For this review, take the finished solid that the model builds, in its own axes (mm). A direction names the side the tool comes from. Coordinates: 2 decimals unless noted, no trailing zeros. Loops run counter-clockwise (first coordinate to the right, second up) from the corner with the lowest first, then second, coordinate; pieces in that order, holes last.
```python
from build123d import *

# Parameters (mm, degrees)
CLAMP_DEPTH      = 8
SKETCH2_R        = 2.1
SCREW_HOLE_DEPTH = 31.055157627


with BuildPart() as part:
    # Sketch1 → Clamp (new body)
    with BuildSketch(Plane.XY):
        with BuildLine():
            Line((-6.631553363, 7.75), (6.631553363, 7.75))
            ThreePointArc((6.631553363, 7.75), (9.265037623, 4.266037723), (10.2, 0))
            Line((10.2, 0), (10.2, -10.5))
            Line((10.2, -10.5), (22.5, -10.5))
            Line((22.5, -10.5), (22.5, -7.5))
            Line((22.5, -7.5), (13, -7.5))
            Line((13, -7.5), (13, 0))
            ThreePointArc((13, 0), (11.489805152, 6.081478239), (7.310095759, 10.75))
            Line((7.310095759, 10.75), (-7.310095759, 10.75))
            ThreePointArc((-7.310095759, 10.75), (-11.489805152, 6.081478239), (-13, 0))
            Line((-13, 0), (-13, -7.5))
            Line((-13, -7.5), (-22.5, -7.5))
            Line((-22.5, -7.5), (-22.5, -10.5))
            Line((-22.5, -10.5), (-10.2, -10.5))
            Line((-10.2, -10.5), (-10.2, 0))
            ThreePointArc((-10.2, 0), (-9.265037623, 4.266037723), (-6.631553363, 7.75))
        make_face()
    extrude(amount=CLAMP_DEPTH)

    # Sketch2 → Screw Hole (cut, through all)
    with BuildSketch(Plane(origin=(0, -7.5, 0), x_dir=(1, 0, 0), z_dir=(0, 1, 0))):
        with Locations(Location((-17.75, -4, 0), (0, 0, 270))):
            Circle(SKETCH2_R)
        with Locations(Location((17.75, -4, 0), (0, 0, 270))):
            Circle(SKETCH2_R)
    extrude(amount=-SCREW_HOLE_DEPTH, mode=Mode.SUBTRACT)


solid = part.part
```
Q1. The part is to be moulded in two halves that separate along X. For faces 5 (the face through (11.531, 6.003, 3.944)), 6 (the face through (15, -10.5, 4)), 7 (the face through (-9.29, 4.21, 3.94)), say which applies: +X half, -X half, draft (parallel to the pull), parting line (faces both ways), or undercut.
Q2. Consider section C-C (x = -17.75). State the section outline as (y, z) points, then the cut area to 3 significant figures.
Q3. Consider section B-B (y = -6.75). State the section outline as (x, z) points, then the cut area to 3 significant figures.
Q4. Consider section A-A (z = 4). State the section outline as (x, y) points, then the cut area to 3 significant figures.
Q5. Wall thickness on probe 1 along X at (y, z) = (-9.65, 4); probe 2 along X at (y, z) = (-0.5, 5.5); probe 3 along Y at (x, z) = (-13.5, 7): over which ranges is each line inside the solid? List them lowest first.
Q6. Machinability: for faces 1 (the face through (-15.668, -8.979, 3.727)), 2 (the face through (-10.2, -5, 4)), 3 (the face through (13, -4, 4)), 4 (the face through (-15.6, -7.5, 3.1)), which of the approach directions +Z, -Z, +X, -X, +Y, -Y give a long, thin tool a straight path to every point of the face, cutting with its end or side? Answer none if there is none.
Q7. Consider section D-D (z = 7.5). State the section outline as (x, y) points, then the cut area to 3 significant figures.
Q8. For pin 1 Ø2.5 at (x, z) = (0.5, 5) entering from -Y; pin 2 Ø2.5 at (x, z) = (-18.5, 3) entering from +Y; pin 3 Ø1 at (y, z) = (-6.5, 4.5) entering from +X, all flat-tipped, find the tip position at first contact; note any pin that passes through.
Model answer:
1. face 5: +X half
1. face 6: draft
1. face 7: undercut
2. outline: (-10.5, 0) - (-7.5, 0) - (-7.5, 1.9) - (-10.5, 1.9) - close; (-10.5, 6.1) - (-7.5, 6.1) - (-7.5, 8) - (-10.5, 8) - close
2. area: 11.4 mm2
3. outline: (-13, 0) - (-10.2, 0) - (-10.2, 8) - (-13, 8) - close; (10.2, 0) - (13, 0) - (13, 8) - (10.2, 8) - close
3. area: 44.8 mm2
4. outline: (-22.5, -10.5) - (-19.85, -10.5) - (-19.85, -7.5) - (-22.5, -7.5) - close; (-15.65, -10.5) - (-10.2, -10.5) - (-10.2, 0) arc R10.2 cw to (-6.63, 7.75) - (6.63, 7.75) arc R10.2 cw to (10.2, 0) - (10.2, -10.5) - (15.65, -10.5) - (15.65, -7.5) - (13, -7.5) - (13, 0) arc R13 ccw to (7.31, 10.75) - (-7.31, 10.75) arc R13 ccw to (-13, 0) - (-13, -7.5) - (-15.65, -7.5) - close; (19.85, -10.5) - (22.5, -10.5) - (22.5, -7.5) - (19.85, -7.5) - close
4. area: 193 mm2
5. probe 1: x = -22.5 to -19.85, -15.65 to -10.2, 10.2 to 15.65, 19.85 to 22.5
5. probe 2: x = -13 to -10.2, 10.2 to 13
5. probe 3: y = -10.5 to -7.5
6. face 1: +Y, -Y
6. face 2: +Z, -Z, -Y
6. face 3: +Z, -Z, +X, +Y
6. face 4: +Z, -Z, -X, +Y
7. outline: (-22.5, -10.5) - (-10.2, -10.5) - (-10.2, 0) arc R10.2 cw to (-6.63, 7.75) - (6.63, 7.75) arc R10.2 cw to (10.2, 0) - (10.2, -10.5) - (22.5, -10.5) - (22.5, -7.5) - (13, -7.5) - (13, 0) arc R13 ccw to (7.31, 10.75) - (-7.31, 10.75) arc R13 ccw to (-13, 0) - (-13, -7.5) - (-22.5, -7.5) - close
7. area: 218 mm2
8. pin 1: stops at y = 7.75
8. pin 2: stops at y = -7.5
8. pin 3: stops at x = 13
